The drawing under review shows one solid part. Ordinate dimensions are in mm from its lowest x, y, z. Coordinates: 2 decimals unless noted, no trailing zeros. Order: outer loops, then holes, each group sorted by start corner. A loop starts at its lowest first (then second) coordinate and runs counter-clockwise, first axis right, second up. Notation, with made-up numbers: M 35,-35 L 60,-35 A28 ccw 60,-5 Z; hole C -37,59.25 d5. An arc over 180 degrees is marked long. Answer as a JSON object with one key per item and string values.
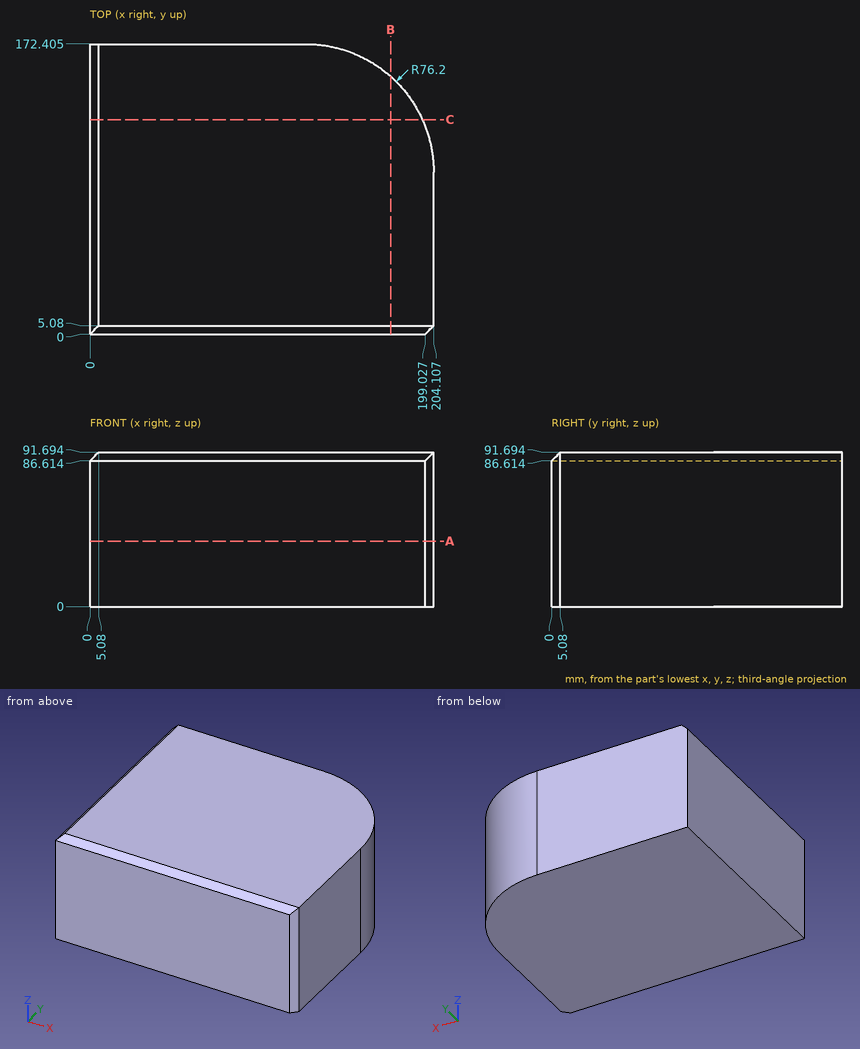
1) To check wall thickness, follow L1, parallel to X at y = 134, z = 14.5; L2, parallel to X at y = 113, z = 58; L3, parallel to Y at x = 157.5, z = 27.5. State the ranges of each line that lie inside material, in increasing order.
Taken from the geometry:
{"L1": "x = 0 to 194.07", "L2": "x = 0 to 202.23", "L3": "y = 0 to 166.42"}
2) Add section A-A (z = 39). State the section outline as (x, y) points (1 decimal).
Taken from the geometry:
{"outline": "M 0,0 L 199,0 L 204.1,5.1 L 204.1,96.2 A76.2 ccw 127.9,172.4 L 0,172.4 Z"}
3) Add section B-B (x = 178.5). State the section outline as (y, z) points (1 decimal), and give its area (3 significant figures).
Taken from the geometry:
{"outline": "M 0,0 L 153.2,0 L 153.2,91.7 L 5.1,91.7 L 0,86.6 Z", "area": "14,000 mm2"}
4) Add section C-C (y = 127.5). State the section outline as (x, z) points, and give its area (3 significant figures).
Taken from the geometry:
{"outline": "M 0,0 L 197.38,0 L 197.38,91.69 L 5.08,91.69 L 0,86.61 Z", "area": "18,100 mm2"}
